from build123d import *

# Parameters (mm, degrees)
F0_W     = 750
F0_H     = 50
F1_DEPTH = 20
F2_W     = 50
F2_H     = 660
F3_DEPTH = 10
F5_DEPTH = 5
F9_DEPTH = 5


with BuildPart() as f1:
    # F0 (on Top) → F1 (new body)
    with BuildSketch(Plane.XY):
        with Locations((0, -305)):
            Rectangle(F0_W, F0_H)
    extrude(amount=F1_DEPTH)


with BuildPart() as f1b:
    # F0 (on Top) → F1, piece 2 (new body)
    with BuildSketch(Plane.XY):
        with Locations((0, 305)):
            Rectangle(F0_W, F0_H)
    extrude(amount=F1_DEPTH)


with BuildPart() as f3:
    # F2 (on face) → F3 (new body)
    with BuildSketch(Plane.XY.offset(20)):
        with Locations((-337.1062517166, 0)):
            Rectangle(F2_W, F2_H)
    extrude(amount=F3_DEPTH)


with BuildPart() as f3b:
    # F2 (on face) → F3, piece 2 (new body)
    with BuildSketch(Plane.XY.offset(20)):
        with Locations((337.1062517166, 0)):
            Rectangle(F2_W, F2_H)
    extrude(amount=F3_DEPTH)


with BuildPart() as f3c:
    # F2 (on face) → F3, piece 3 (new body)
    with BuildSketch(Plane.XY.offset(20)):
        with Locations((-130.3327232599, 0)):
            Rectangle(F2_W, F2_H)
    extrude(amount=F3_DEPTH)


with BuildPart() as f3d:
    # F2 (on face) → F3, piece 4 (new body)
    with BuildSketch(Plane.XY.offset(20)):
        with Locations((130.3327232599, 0)):
            Rectangle(F2_W, F2_H)
    extrude(amount=F3_DEPTH)


with BuildPart() as f5:
    # F4 (on face) → F5 (new body)
    with BuildSketch(Plane.XY.offset(20)):
        Polygon((-296.1573302746, -263.5724842548), (-300, -280), (-280, -280), (-283.8426697254, -263.5724842548), (-287.3255479336, -257.0246756077), (-290, -257.0246756077), (-292.6744520664, -257.0246756077), align=None)
        Polygon((-280, -280), (-300, -280), (-325, -280), (-325, -295), (265, -295), (265, -280), (240, -280), (220, -280), (200, -280), (180, -280), (160, -280), (140, -280), (120, -280), (100, -280), (80, -280), (60, -280), (40, -280), (20, -280), (0, -280), (-20, -280), (-40, -280), (-60, -280), (-80, -280), (-100, -280), (-120, -280), (-140, -280), (-160, -280), (-180, -280), (-200, -280), (-220, -280), (-240, -280), (-260, -280), align=None)
        Polygon((-256.1573302746, -263.5724842548), (-260, -280), (-240, -280), (-243.8426697254, -263.5724842548), (-247.3255479336, -257.0246756077), (-250, -257.0246756077), (-252.6744520664, -257.0246756077), align=None)
        Polygon((-216.1573302746, -263.5724842548), (-220, -280), (-200, -280), (-203.8426697254, -263.5724842548), (-207.3255479336, -257.0246756077), (-210, -257.0246756077), (-212.6744520664, -257.0246756077), align=None)
        Polygon((220, -280), (240, -280), (236.1573302746, -263.5724842548), (232.6744520664, -257.0246756077), (230, -257.0246756077), (227.3255479336, -257.0246756077), (223.8426697254, -263.5724842548), align=None)
        Polygon((-176.1573302746, -263.5724842548), (-180, -280), (-160, -280), (-163.8426697254, -263.5724842548), (-167.3255479336, -257.0246756077), (-170, -257.0246756077), (-172.6744520664, -257.0246756077), align=None)
        Polygon((180, -280), (200, -280), (196.1573302746, -263.5724842548), (192.6744520664, -257.0246756077), (190, -257.0246756077), (187.3255479336, -257.0246756077), (183.8426697254, -263.5724842548), align=None)
        Polygon((-136.1573302746, -263.5724842548), (-140, -280), (-120, -280), (-123.8426697254, -263.5724842548), (-127.3255479336, -257.0246756077), (-130, -257.0246756077), (-132.6744520664, -257.0246756077), align=None)
        Polygon((140, -280), (160, -280), (156.1573302746, -263.5724842548), (152.6744520664, -257.0246756077), (150, -257.0246756077), (147.3255479336, -257.0246756077), (143.8426697254, -263.5724842548), align=None)
        Polygon((-96.1573302746, -263.5724842548), (-100, -280), (-80, -280), (-83.8426697254, -263.5724842548), (-87.3255479336, -257.0246756077), (-90, -257.0246756077), (-92.6744520664, -257.0246756077), align=None)
        Polygon((100, -280), (120, -280), (116.1573302746, -263.5724842548), (112.6744520664, -257.0246756077), (110, -257.0246756077), (107.3255479336, -257.0246756077), (103.8426697254, -263.5724842548), align=None)
        Polygon((-56.1573302746, -263.5724842548), (-60, -280), (-40, -280), (-43.8426697254, -263.5724842548), (-47.3255479336, -257.0246756077), (-50, -257.0246756077), (-52.6744520664, -257.0246756077), align=None)
        Polygon((60, -280), (80, -280), (76.1573302746, -263.5724842548), (72.6744520664, -257.0246756077), (70, -257.0246756077), (67.3255479336, -257.0246756077), (63.8426697254, -263.5724842548), align=None)
        Polygon((-16.1573302746, -263.5724842548), (-20, -280), (0, -280), (-3.8426697254, -263.5724842548), (-7.3255479336, -257.0246756077), (-10, -257.0246756077), (-12.6744520664, -257.0246756077), align=None)
        Polygon((20, -280), (40, -280), (36.1573302746, -263.5724842548), (32.6744520664, -257.0246756077), (30, -257.0246756077), (27.3255479336, -257.0246756077), (23.8426697254, -263.5724842548), align=None)
    extrude(amount=-F5_DEPTH)

    # F8 (on face) → F9 (join)
    with BuildSketch(Plane.XY.offset(20)):
        Polygon((-280, -280), (-286.9936227798, -249.4549155235), (-293.270021677, -238.5834902525), (-296.9827055931, -238.5834902525), (-305.3558170795, -280), align=None)
    extrude(amount=-F9_DEPTH)


with BuildPart() as f5b:
    # F4 (on face) → F5, piece 2 (new body)
    with BuildSketch(Plane.XY.offset(20)):
        Polygon((-280, 280), (-300, 280), (-296.1573302746, 263.5724842548), (-292.6744520664, 257.0246756077), (-290, 257.0246756077), (-287.3255479336, 257.0246756077), (-283.8426697254, 263.5724842548), align=None)
        Polygon((-325, 280), (-300, 280), (-280, 280), (-260, 280), (-240, 280), (-220, 280), (-200, 280), (-180, 280), (-160, 280), (-140, 280), (-120, 280), (-100, 280), (-80, 280), (-60, 280), (-40, 280), (-20, 280), (0, 280), (20, 280), (40, 280), (60, 280), (80, 280), (100, 280), (120, 280), (140, 280), (160, 280), (180, 280), (200, 280), (220, 280), (240, 280), (265, 280), (265, 305), (-325, 305), align=None)
        Polygon((-240, 280), (-260, 280), (-256.1573302746, 263.5724842548), (-252.6744520664, 257.0246756077), (-250, 257.0246756077), (-247.3255479336, 257.0246756077), (-243.8426697254, 263.5724842548), align=None)
        Polygon((-200, 280), (-220, 280), (-216.1573302746, 263.5724842548), (-212.6744520664, 257.0246756077), (-210, 257.0246756077), (-207.3255479336, 257.0246756077), (-203.8426697254, 263.5724842548), align=None)
        Polygon((236.1573302746, 263.5724842548), (240, 280), (220, 280), (223.8426697254, 263.5724842548), (227.3255479336, 257.0246756077), (230, 257.0246756077), (232.6744520664, 257.0246756077), align=None)
        Polygon((-160, 280), (-180, 280), (-176.1573302746, 263.5724842548), (-172.6744520664, 257.0246756077), (-170, 257.0246756077), (-167.3255479336, 257.0246756077), (-163.8426697254, 263.5724842548), align=None)
        Polygon((196.1573302746, 263.5724842548), (200, 280), (180, 280), (183.8426697254, 263.5724842548), (187.3255479336, 257.0246756077), (190, 257.0246756077), (192.6744520664, 257.0246756077), align=None)
        Polygon((-120, 280), (-140, 280), (-136.1573302746, 263.5724842548), (-132.6744520664, 257.0246756077), (-130, 257.0246756077), (-127.3255479336, 257.0246756077), (-123.8426697254, 263.5724842548), align=None)
        Polygon((156.1573302746, 263.5724842548), (160, 280), (140, 280), (143.8426697254, 263.5724842548), (147.3255479336, 257.0246756077), (150, 257.0246756077), (152.6744520664, 257.0246756077), align=None)
        Polygon((-80, 280), (-100, 280), (-96.1573302746, 263.5724842548), (-92.6744520664, 257.0246756077), (-90, 257.0246756077), (-87.3255479336, 257.0246756077), (-83.8426697254, 263.5724842548), align=None)
        Polygon((116.1573302746, 263.5724842548), (120, 280), (100, 280), (103.8426697254, 263.5724842548), (107.3255479336, 257.0246756077), (110, 257.0246756077), (112.6744520664, 257.0246756077), align=None)
        Polygon((-40, 280), (-60, 280), (-56.1573302746, 263.5724842548), (-52.6744520664, 257.0246756077), (-50, 257.0246756077), (-47.3255479336, 257.0246756077), (-43.8426697254, 263.5724842548), align=None)
        Polygon((76.1573302746, 263.5724842548), (80, 280), (60, 280), (63.8426697254, 263.5724842548), (67.3255479336, 257.0246756077), (70, 257.0246756077), (72.6744520664, 257.0246756077), align=None)
        Polygon((0, 280), (-20, 280), (-16.1573302746, 263.5724842548), (-12.6744520664, 257.0246756077), (-10, 257.0246756077), (-7.3255479336, 257.0246756077), (-3.8426697254, 263.5724842548), align=None)
        Polygon((36.1573302746, 263.5724842548), (40, 280), (20, 280), (23.8426697254, 263.5724842548), (27.3255479336, 257.0246756077), (30, 257.0246756077), (32.6744520664, 257.0246756077), align=None)
    extrude(amount=-F5_DEPTH)


solid = f5.part
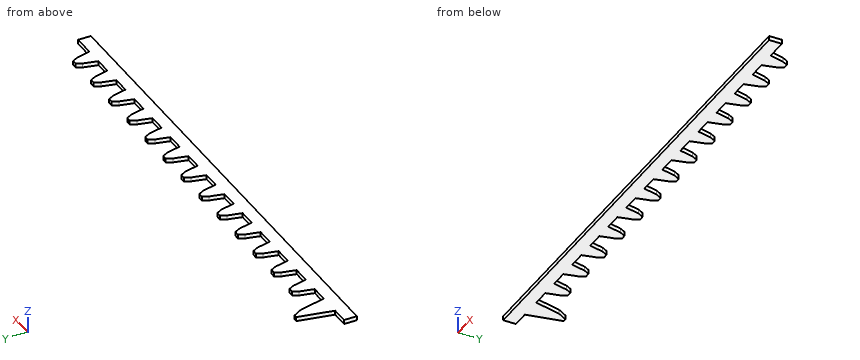
Input: part model. Units: mm. Frame: model coordinates. Round coordinates to 2 decimals unless told otherwise and drop trailing zeros. Loops run counter-clockwise (first coordinate to the right, second up) from the corner with the lowest first, then second, coordinate; pieces in that order, holes last. Notation, with made-up numbers: M 60.25,18 L 77.25,18 A5 cw 77.25,24 Z; hole C 44.25,18.25 d11. An arc over 180 degrees is marked long. Answer as CSV lines item,"result". Start each with the question number.
(1) Section B-B, the plane y = -244.5. Output: boundary loops of the cut face in (x, z), plus the area to 3 significant figures.
(2) Line query: line 1 (Y direction, x = -222.5, z = 15.8); line 2 (Y direction, x = -89.5, z = 18.1); line 3 (X direction, y = -251.5, z = 15.7). Output: solid intervals per line, ascending. Write a range as [from, to].
(3) Section A-A, the plane x = -111. Output: boundary loops of the cut face in (y, z).
(4) First-contact query: pin 1 (1.5 mm diameter, centred on x = 167, z = 18.5, fed in from +Y); pin 2 (1.5 mm diameter, centred on x = 69.5, z = 16.5, fed in from +Y); pin 3 (2 mm diameter, centred on y = -264.5, z = 19.5, fed in from -X). Flat tips, straight axial feed; report the tip coordinate or a pass-through.
Values found:
1,outline,"M -298.18,15 L -289.85,15 L -289.85,20 L -298.18,20 Z"
1,area,"41.6 mm²"
2,line 1,"y = [-295, -280]"
2,line 2,"y = [-295, -257.02]"
2,line 3,"x = [-299.59, -286.53]"
3,outline,"M -295,15 L -280,15 L -280,20 L -295,20 Z"
4,pin 1,"stops at y = -280"
4,pin 2,"stops at y = -257.02"
4,pin 3,"stops at x = -302.42"
